Job drawing, mm, ordinate dimensions from the low corner. One solid piece. A direction names the side the tool comes from. Round coordinates to 2 decimals unless told otherwise and drop trailing zeros. Write each loop counter-clockwise with the first axis right and the second up, starting at its lowest first coordinate (ties: lowest second). Pieces come first, ordered by that corner, then holes.
1) Pull direction X, two halves, no side cores. Call the marked faces 1, 2, 3 and 4: +X half, -X half, draft (parallel to the pull), parting line (faces both ways), or undercut.
2) Saw through at C-C (y = 13.5). Write the cut outline in (x, z), plus the area to 3 significant figures.
3) Saw through at D-D (y = 5). Write the cut outline in (x, z).
4) Flat gauge pins, fed straight in: pin 1 (5 mm diameter, centred on x = 8, y = 16.5, fed in from +Z) (1 decimal); pin 2 (4 mm diameter, centred on y = 17.5, z = 12.5, fed in from +X); pin 3 (12 mm diameter, centred on y = 7, z = 5, fed in from +X). Where does each tip first touch, or does it go through?
5) Wall check: probe 1 along Z at (x, y) = (18, 4.75); probe 2 along Z at (x, y) = (18, 8.25); probe 3 along X at (y, z) = (17.5, 21) (1 decimal). Give the ranges that are in metal, low to high.
6) Which spindle directions (+Z, -Z, +X, -X, +Y, -Y) get a long thin tool onto all of the face, cutting with end or side? Do the marked faces 5 and 6. Say none if no direction does.
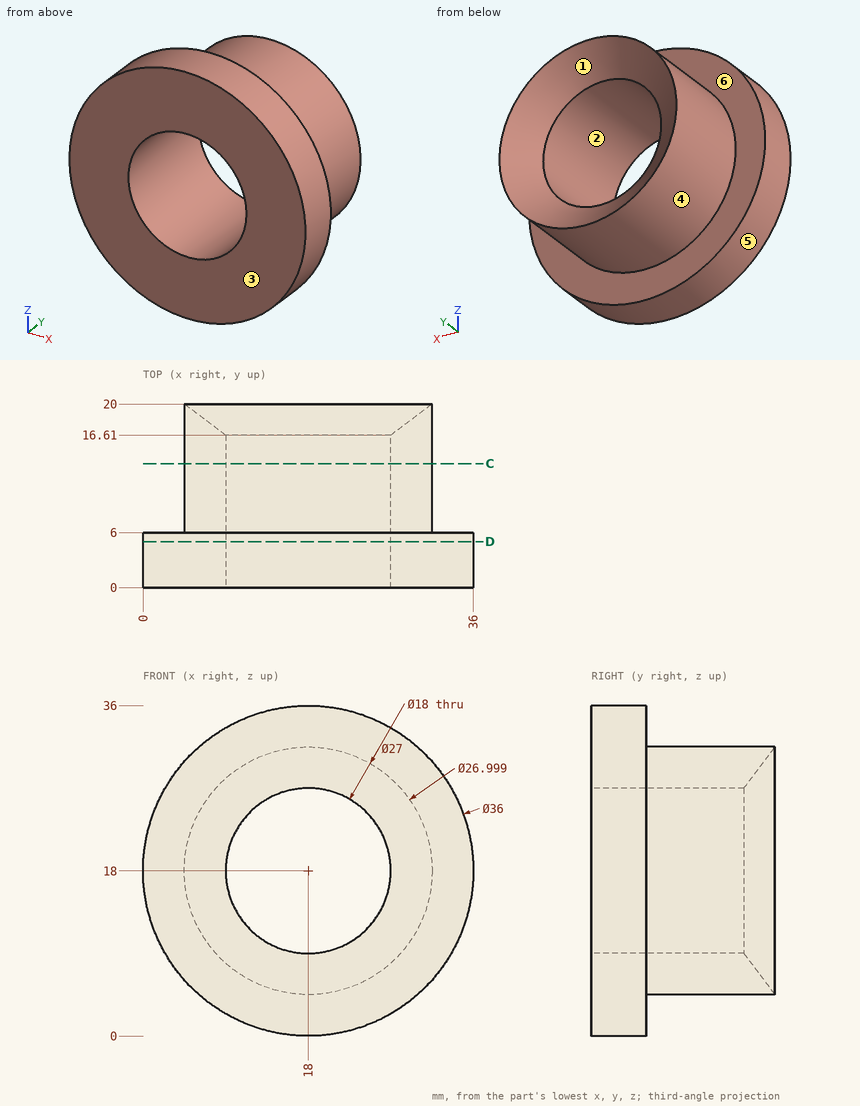
Evaluation:
1. face 1: undercut
1. face 2: undercut
1. face 3: draft
1. face 4: parting line
2. outline: circle Ø27 at (18, 18); hole circle Ø18 at (18, 18)
2. area: 318 mm2
3. outline: circle Ø36 at (18, 18); hole circle Ø18 at (18, 18)
4. pin 1: stops at z = 29.2
4. pin 2: stops at x = 31.04
4. pin 3: stops at x = 34.55
5. probe 1: z = 0 to 9, 27 to 36
5. probe 2: z = 4.5 to 9, 27 to 31.5
5. probe 3: x = 4.8 to 8.3, 27.7 to 31.2
6. face 5: +Y, -Y
6. face 6: +Y
